Design review of the part built by this model. Coordinates are the model's own, in mm. Face numbers are marked on the shaded views. A direction names the side the tool comes from. Coordinates: 2 decimals unless noted, no trailing zeros. Write each loop counter-clockwise with the first axis right and the second up, starting at its lowest first coordinate (ties: lowest second). Pieces come first, ordered by that corner, then holes. Notation, with made-up numbers: M -26.75,-21.75 L -7.75,-21.75 A34 ccw -7.75,10.25 Z; hole C -5.75,77.5 d8. An arc over 180 degrees is marked long. One line per question, with ' | ' between items.
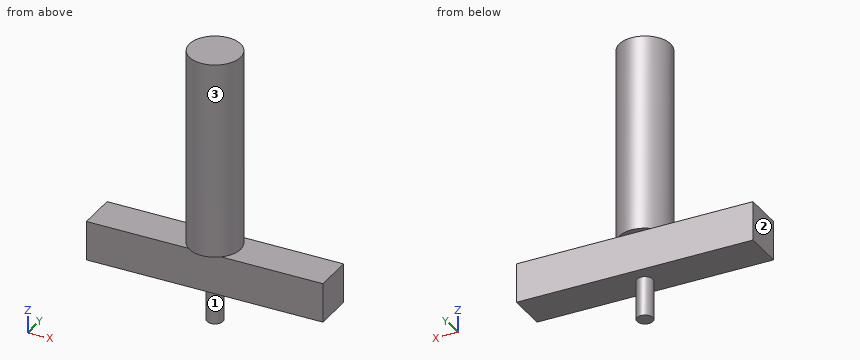
from build123d import *

# Parameters (mm, degrees)
F1_R     = 6.5
F3_W     = 60
F3_H     = 10
F4_DEPTH = 10
F5_R     = 2
F6_DEPTH = 20


with BuildPart() as f2:
    # F2: sweep along a path in F0
    with BuildLine(Plane.XZ) as f2_path:
        Line((0, 50), (0, 0))
    # F1 (on Top) → F2 (sweep)
    with BuildSketch(Plane.XY):
        Circle(F1_R)
    sweep(path=f2_path.line)

    # F3 (on Top) → F4 (join)
    with BuildSketch(Plane.XY):
        Rectangle(F3_W, F3_H)
    extrude(amount=-F4_DEPTH)

    # F5 (on Top) → F6 (join)
    with BuildSketch(Plane.XY):
        Circle(F5_R)
    extrude(amount=-F6_DEPTH)


solid = f2.part
1. Take a section at D-D (y = -3.5). Write out the cut boundary in (x, z).
Answer sheet:
outline: M -30,-10 L 30,-10 L 30,0 L 5.48,0 L 5.48,50 L -5.48,50 L -5.48,0 L -30,0 Z
2. Take a section at C-C (z = 27.5). Write out the cut boundary in (x, y).
Answer sheet:
outline: C 0,0 d13
3. To check wall thickness, follow line 1 along X through (y, z) = (-0.25, 15.5); line 2 along Y through (x, z) = (8.5, -2); line 3 along Z through (x, y) = (6, -3.5). State the ranges of each line that lie inside material, in increasing order. Write a range as [from, to].
Answer sheet:
line 1: [-6.5, 6.5] | line 2: [-5, 5] | line 3: [-10, 0]
4. Take a section at B-B (y = 0). Write out the cut boundary in (x, z), then the cut area to 3 significant figures.
Answer sheet:
outline: M -30,-10 L -2,-10 L -2,-20 L 2,-20 L 2,-10 L 30,-10 L 30,0 L 6.5,0 L 6.5,50 L -6.5,50 L -6.5,0 L -30,0 Z | area: 1,290 mm^2
5. Tool access review of the marked faces 1, 2 and 3: name each direction out of +Z, -Z, +X, -X, +Y, -Y from which nothing blocks a thin tool from reaching the whole face with its end or side.
Answer sheet:
face 1: -Z | face 2: +Z, -Z, -X, +Y, -Y | face 3: +Z
6. Insertion check: pin 1 Ø5 at (x, y) = (4.5, 1) entering from -Z; pin 2 Ø4 at (y, z) = (-0.5, 41) entering from +X; pin 3 Ø6 at (x, z) = (16.5, -6) entering from -Y. Each pin has a flat end and moves straight along its axis. Give the tip position at first contact, or say it passes through.
Answer sheet:
pin 1: z = -10 | pin 2: x = 6.5 | pin 3: y = -5
7. Take a section at A-A (x = 0). Write out the cut boundary in (y, z), then the cut area to 3 significant figures.
Answer sheet:
outline: M -6.5,0 L -5,0 L -5,-10 L -2,-10 L -2,-20 L 2,-20 L 2,-10 L 5,-10 L 5,0 L 6.5,0 L 6.5,50 L -6.5,50 Z | area: 790 mm^2
